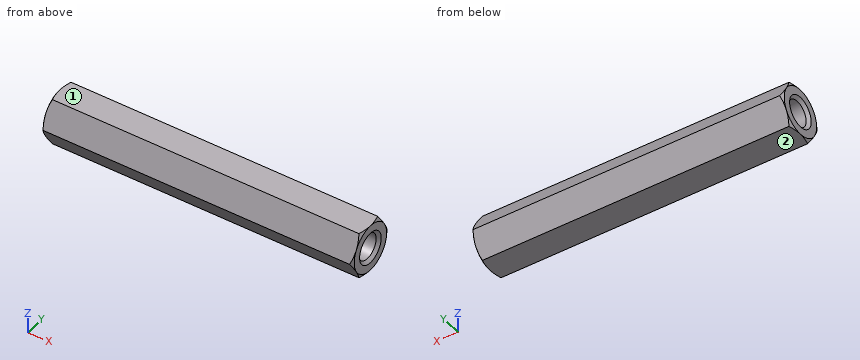
Autodesk Inventor part; units mm, degrees
ref_plane "C3_XY" through (39.5, 0, 0) normal (-1, 0, 0) x (0, 0, -1)
ref_plane "C3_YZ" through (39.5, 0, 0) normal (0, 0, -1) x (0, -1, 0)
ref_plane "C3_ZX" through (39.5, 0, 0) normal (0, -1, 0) x (-1, 0, 0)
sketch "Sketch_1" plane through (0, 0, 0) normal (0, 0, 1) x (1, 0, 0)
  line L0 (39.5, 0) -> (0, 0)
  line L1 (0, 0) -> (0, 3)
  line L2 (0, 3) -> (0.5485, 3.95)
  line L3 (0.5485, 3.95) -> (38.9515, 3.95)
  line L4 (38.9515, 3.95) -> (39.5, 3)
  line L5 (39.5, 3) -> (39.5, 0)
  line L6 (39.5, 0) -> (0, 0)
revolve "Revolution1" add sketch "Sketch_1" angle 360 about axis through (39.5, 0, 0) along (1, 0, 0)
sketch "Sketch_2" plane through (0, 0, 0) normal (1, 0, 0) x (0, 1, 0)
  line L0 (6, 6) -> (-6, 6)
  line L1 (-6, 6) -> (-6, -6)
  line L2 (-6, -6) -> (6, -6)
  line L3 (6, -6) -> (6, 6)
  line L4 (-1.7321, 3) -> (-3.4641, 0)
  line L5 (-3.4641, 0) -> (-1.7321, -3)
  line L6 (-1.7321, -3) -> (1.7321, -3)
  line L7 (1.7321, -3) -> (3.4641, 0)
  line L8 (3.4641, 0) -> (1.7321, 3)
  line L9 (1.7321, 3) -> (-1.7321, 3)
extrude "Extrusion1" cut sketch "Sketch_2" along normal blind 39.5
sketch "Sketch3" plane through (0, 0, 0) normal (-1, 0, 0) x (0, 0, 1)
  point P0 (0, 0)
hole "Hole1" at (0, 0, 0) direction (1, 0, 0) diameter 3.242 depth 11.0641 tip angle 120 countersink diameter 4 countersink angle 90
sketch "Sketch4" plane through (39.5, 0, 0) normal (1, 0, 0) x (0, 0, -1)
  point P0 (0, 0)
hole "Hole2" at (39.5, 0, 0) direction (-1, 0, 0) diameter 3.242 depth 11.0641 tip angle 120 countersink diameter 4 countersink angle 90
ref_plane "C3_XY" through (39.5, 0, 0) normal (-1, 0, 0) x (0, 0, -1)
ref_plane "C3_YZ" through (39.5, 0, 0) normal (0, 0, -1) x (0, -1, 0)
ref_plane "C3_ZX" through (39.5, 0, 0) normal (0, -1, 0) x (-1, 0, 0)
properties part number "SLSBF6-39.5-M4-N4"
Can you work these out from the model? Positions are in its coordinate system, mm. Face numbers are marked on the shaded views. Round coordinates to 2 decimals unless told otherwise and drop trailing zeros. Order: outer loops, then holes, each group sorted by start corner. A loop starts at its lowest first (then second) coordinate and runs counter-clockwise, first axis right, second up. Notation, with made-up numbers: (-39.75, -31.5) - (-13.75, -31.5) arc R22 cw to (-13.75, -13.5) - close; hole circle Ø10 at (87, 52.25). An arc over 180 degrees is marked (long way). Answer in a Markdown table with one row per item.
(1) Suppose I cut it at B-B, the plane x = 17. Please give me the cut outline in (y, z), plus the area to 3 significant figures.
From the geometry:
| item | result |
|---|---|
| outline | (-3.46, 0) - (-1.73, -3) - (1.73, -3) - (3.46, 0) - (1.73, 3) - (-1.73, 3) - close |
| area | 31.2 mm2 |
(2) If we mould it in two halves opening along Z, with no side actions, what happens to the marked faces 1 and 2? For each: released by +Z, released by -Z, zero draft, split by the parting line, or undercut.
From the geometry:
| item | result |
|---|---|
| face 1 | released by +Z |
| face 2 | released by -Z |
(3) For P1, Ø1, axis at y = 1.5, z = 2, coming from the -X side; P2, Ø3, axis at y = 0, z = 0, coming from the -X side; P3, Ø3, axis at x = 11.5, z = 2, coming from the +Y side; P4, Ø2.5, axis at y = 0, z = 0, coming from the -X side, each with a flat end and sliding along its axis, tell me the tip position at first contact or that it passes through.
From the geometry:
| item | result |
|---|---|
| P1 | stops at x = 0 |
| P2 | stops at x = 11.13 |
| P3 | stops at y = 3.18 |
| P4 | stops at x = 11.28 |
(4) Suppose I cut it at A-A, the plane x = 33. Please give me the cut outline in (y, z).
From the geometry:
| item | result |
|---|---|
| outline | (-3.46, 0) - (-1.73, -3) - (1.73, -3) - (3.46, 0) - (1.73, 3) - (-1.73, 3) - close; hole circle Ø3.24 at (0, 0) |
(5) Please list where these lines run through material, in increasing order: L1, parallel to Z at x = 36, y = 0; L2, parallel to Y at x = 28, z = 0.6; L3, parallel to Z at x = 11.5, y = -0.25. Write a range as from..to.
From the geometry:
| item | result |
|---|---|
| L1 | z = -3..-1.62, 1.62..3 |
| L2 | y = -3.12..-0.62, 0.62..3.12 |
| L3 | z = -3..-0.83, 0.83..3 |
